from build123d import *

# Parameters (mm, degrees)
F1_DEPTH  = 127
F2_DEPTH  = 114.3
F3_DEPTH  = 88.9
F6_DEPTH  = 76.2
F8_W      = 64.8522339761
F8_H      = 74.062012136
F9_DEPTH  = 38.1
F10_T     = -2.54
F11_W     = 125.4833117127
F11_H     = 19.5707902312
F12_DEPTH = 101.6
F14_W     = 127
F14_H     = 100.4699997724
F15_DEPTH = 127


# Not quite as in the source:
# - a shell that OpenCascade refuses in one call is made with other operations: the cavity is built on its own and cut out


with BuildPart() as f1:
    # F0 (on Top) → F1 (new body)
    with BuildSketch(Plane.XY):
        Polygon((27.6681821086, 78.8052295411), (-99.3318178914, 78.8052295411), (-99.3318178914, -22.7947704589), (-35.8318178914, -22.7947704589), (27.6681821086, -22.7947704589), align=None)
    extrude(amount=F1_DEPTH)

    # F0 (on Top) → F2 (join)
    with BuildSketch(Plane.XY):
        Polygon((27.6681821086, -124.3947704589), (27.6681821086, -22.7947704589), (-35.8318178914, -22.7947704589), (-35.8318178914, -95.8602428436), (-35.8318178914, -124.3947704589), align=None)
    extrude(amount=F2_DEPTH)

    # F0 (on Top) → F3 (join)
    with BuildSketch(Plane.XY):
        Polygon((-35.8318178914, -124.3947704589), (-35.8318178914, -95.8602428436), (-69.7213560343, -95.8602428436), (-69.7213560343, -85.9395861626), (-69.7213560343, -78.0614241958), (-50.7554039359, -78.0614241958), (-50.7554039359, -43.129093945), (-99.3318178914, -43.129093945), (-99.3318178914, -124.3947704589), align=None)
    extrude(amount=F3_DEPTH)

    # F5 (on offset) → F6 (join)
    with BuildSketch(Plane.XZ.offset(-95.25)):
        Polygon((-109.9954843521, 12.5446757302), (27.7675427496, 12.5446757302), (39.663515985, 12.1609345078), (39.663515985, 116.1547526717), (-109.9954843521, 116.1547526717), align=None)
    extrude(amount=F6_DEPTH)

    # F8 (on offset) → F9 (join)
    with BuildSketch(Plane.YZ.offset(61.214)):
        with Locations((16.1268953234, 56.4830191433)):
            Rectangle(F8_W, F8_H)
    extrude(amount=-F9_DEPTH)

    # F10: a shell. OpenCascade refuses it in one call, so the cavity is built on its own and cut out:
    # the body offset inwards by the wall thickness, plus a prism from it out through each open face.
    f10_core = offset(f1.part, amount=F10_T, kind=Kind.INTERSECTION, mode=Mode.PRIVATE)
    f10_exits = [f10_core.faces().sort_by_distance(p)[0] for p in [
        (-52.776587, -98.400243, 44.45),
    ]]
    add(f10_core, mode=Mode.SUBTRACT)
    extrude(f10_exits, amount=-F10_T, mode=Mode.SUBTRACT)

    # F11 (on offset) → F12 (join)
    with BuildSketch(Plane.XZ.offset(-95.25)):
        with Locations((-39.538461715, 90.2522318065)):
            Rectangle(F11_W, F11_H)
    extrude(amount=-F12_DEPTH)

    # F14 (on offset) → F15 (join)
    with BuildSketch(Plane.XZ.offset(-196.85)):
        with Locations((-39.6279752942, 50.2349998862)):
            Rectangle(F14_W, F14_H)
    extrude(amount=-F15_DEPTH)


solid = f1.part
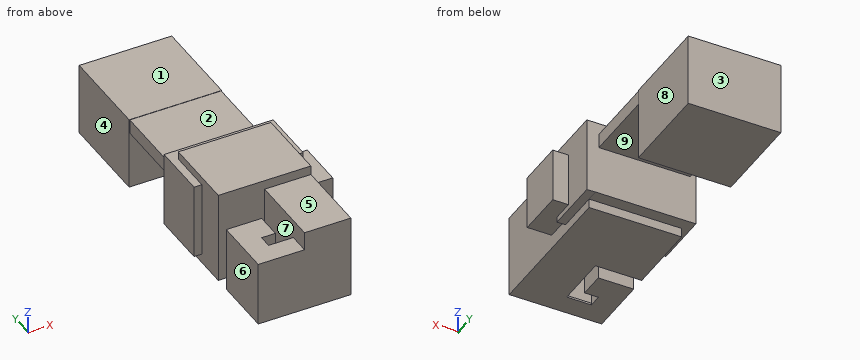
Design review of the part built by this model. Coordinates are the model's own, in mm. Face numbers are marked on the shaded views. A direction names the side the tool comes from. Round coordinates to 2 decimals unless told otherwise and drop trailing zeros. Order: outer loops, then holes, each group sorted by start corner. A loop starts at its lowest first (then second) coordinate and runs counter-clockwise, first axis right, second up.
1) Consider section A-A (y = -51.5). State the section outline as (x, z) points, plus the area to 3 significant figures.
The answers:
outline: (-99.33, 0) - (-50.76, 0) - (-50.76, 88.9) - (-99.33, 88.9) - close; (-35.83, 0) - (27.67, 0) - (27.67, 114.3) - (-35.83, 114.3) - close; hole (-96.79, 2.54) - (-53.3, 2.54) - (-53.3, 86.36) - (-96.79, 86.36) - close; hole (-33.29, 2.54) - (25.13, 2.54) - (25.13, 111.76) - (-33.29, 111.76) - close
area: 1,550 mm2
2) Machinability: for the marked faces 1, 2, 3, 4 and 5, which of the approach directions +Z, -Z, +X, -X, +Y, -Y give a long, thin tool a straight path to every point of the face, cutting with its end or side? Answer none if there is none.
The answers:
face 1: +Z, +X, -X, +Y
face 2: +Z, +X, -X
face 3: +Z, -Z, +X, -X, +Y
face 4: +Z, -Z, -X, +Y
face 5: +Z, +X, -X, -Y
3) For L1, parallel to Y at x = -25, z = 36; L2, parallel to Y at x = -47, z = 84.5; L3, parallel to X at y = -56.5, z = 51.5, list the stretches that pass through material, from the lowest coordinate up.
The answers:
L1: y = -124.39 to -121.85, 92.71 to 95.25, 196.85 to 323.85
L2: y = -124.39 to -121.85, -22.79 to -20.25, 92.71 to 323.85
L3: x = -99.33 to -96.79, -53.3 to -50.76, -35.83 to -33.29, 25.13 to 27.67
4) Clearance check with flat-ended pins moving along their axes: pin 1 Ø10 at (y, z) = (-15.5, 61) entering from -X; pin 2 Ø5 at (x, z) = (-29, 114) entering from +Y; pin 3 Ø5.5 at (x, z) = (-66, 118) entering from -Y. State where each tip first meets the part, or that it passes through.
The answers:
pin 1: stops at x = -99.33
pin 2: stops at y = 95.25
pin 3: stops at y = -22.79
5) Draft analysis for pull direction X (two halves, no side actions). For the marked faces 6, 7, 8 and 9, state which applies: released by +X, released by -X, zero draft, split by the parting line, or undercut.
The answers:
face 6: released by -X
face 7: undercut
face 8: released by +X
face 9: zero draft
6) Consider section D-D (y = 59.5). State the section outline as (x, z) points, plus the area to 3 significant figures.
The answers:
outline: (-110, 12.54) - (-99.33, 12.54) - (-99.33, 0) - (27.67, 0) - (27.67, 12.54) - (27.77, 12.54) - (39.66, 12.16) - (39.66, 116.15) - (27.67, 116.15) - (27.67, 127) - (-99.33, 127) - (-99.33, 116.15) - (-110, 116.15) - close; hole (-107.46, 15.08) - (-96.79, 15.08) - (-96.79, 2.54) - (25.13, 2.54) - (25.13, 15.08) - (27.81, 15.08) - (37.12, 14.78) - (37.12, 113.61) - (25.13, 113.61) - (25.13, 124.46) - (-96.79, 124.46) - (-96.79, 113.61) - (-107.46, 113.61) - close
area: 1,380 mm2
7) Consider section B-B (x = -89). Count the separate pieces of the cut face and the enclosed holes in it, plus the area to 3 significant figures.
The answers:
separate pieces: 2
enclosed holes: 2
area: 16,800 mm2
